```python
from build123d import *

# Parameters (mm, degrees)
F0_R     = 23.495
F0_R_2   = 19.05
F1_DEPTH = 6.35
F2_DEPTH = 149.86
F4_D     = 3.4544
F4_DEPTH = 12.7
F4_TIP   = 1.0378064612
F7_R     = 11.90625
F8_DEPTH = 0.381


with BuildPart() as f1:
    # F0 (on Top) → F1 (new body)
    with BuildSketch(Plane.XY):
        Circle(F0_R)
        Circle(F0_R_2, mode=Mode.SUBTRACT)
    extrude(amount=F1_DEPTH)

    # F0 (on Top) → F2 (join)
    with BuildSketch(Plane.XY):
        Circle(F0_R_2)
    extrude(amount=F2_DEPTH)

    # F4
    with Locations(Plane.XY.offset(149.86)):
        with Locations((0, 0)):
            Hole(F4_D / 2, depth=F4_DEPTH)
            with Locations((0, 0, -(F4_DEPTH + F4_TIP / 2))):  # 118° drill point
                Cone(0, F4_D / 2, F4_TIP, mode=Mode.SUBTRACT)


with BuildPart() as f5_1:
    # F5: copy of F1
    add(f1.part)


with BuildPart() as f1_1:
    add(f1.part)

    # F7 (on face) → F8 (cut)
    with BuildSketch(Plane(origin=(0, 0, 0), x_dir=(1, 0, 0), z_dir=(0, 0, -1))):
        Circle(F7_R)
    extrude(amount=-F8_DEPTH, mode=Mode.SUBTRACT)


solid = f1_1.part
```
Model file for the job. Use its own axes, mm. A direction names the side the tool comes from. Coordinates: 2 decimals unless noted, no trailing zeros. Order: outer loops, then holes, each group sorted by start corner. A loop starts at its lowest first (then second) coordinate and runs counter-clockwise, first axis right, second up. Notation, with made-up numbers: (38, 75) -> (60, 75) arc R4 ccw to (60, 79) -> close; hole circle Ø9 at (68, 29). An arc over 180 degrees is marked (long way). Answer as a JSON object with one key per item and string values. Group by question number.
1) Cut at A-A, the plane y = 8.5. Write the cut outline in (x, z).
2) Drill centre lines: L1, parallel to Y at x = 0, z = 144; L2, parallel to Y at x = 0, z = 0.1 (3 decimals); L3, parallel to Z at x = 19.5, y = -6. Where is each one in solid material? Low to high.
3) Pull direction X, two halves, no side cores. Call faces 4 (the face through (-15.12, -11.59, 77.1)), 5 (the face through (0, 0, 0.381)), 6 (the face through (-11, 6, 0)): +X half, -X half, draft (parallel to the pull), parting line (faces both ways), or undercut.
4) Which spindle directions (+Z, -Z, +X, -X, +Y, -Y) get a long thin tool onto all of the face, cutting with end or side? Do faces 1 (the face through (-5.093, -22.936, 3.131)), 2 (the face through (-0.1, 19.3, 6.35)), 3 (the face through (-9.45, 7.24, 0.19)). Say none if no direction does.
5) Cut at C-C, the plane z = 35. Write the cut outline in (x, y).
6) Flat gauge pins, fed straight in: pin 1 (5 mm diameter, centred on y = -14.5, z = 89.5, fed in from +X); pin 2 (5 mm diameter, centred on x = 9.5, z = 33, fed in from -Y); pin 3 (3 mm diameter, centred on y = 14.5, z = 122, fed in from +X). Where does each tip first touch, or does it go through?
7) Cut at D-D, the plane y = 14.5. Write the cut outline in (x, z), then the cut area to 3 significant figures.
8) Cut at B-B, the plane x = -14. Write the cut outline in (y, z).
Check values:
{
 "1": {"outline": "(-21.9, 0) -> (-8.34, 0) -> (-8.34, 0.38) -> (8.34, 0.38) -> (8.34, 0) -> (21.9, 0) -> (21.9, 6.35) -> (17.05, 6.35) -> (17.05, 149.86) -> (-17.05, 149.86) -> (-17.05, 6.35) -> (-21.9, 6.35) -> close"},
 "2": {"L1": "y = -19.05 to -1.73, 1.73 to 19.05", "L2": "y = -23.495 to -11.906, 11.906 to 23.495", "L3": "z = 0 to 6.35"},
 "3": {"face 4": "parting line", "face 5": "undercut", "face 6": "draft"},
 "4": {"face 1": "+Z, -Z", "face 2": "+Z", "face 3": "-Z"},
 "5": {"outline": "circle Ø38.1 at (0, 0)"},
 "6": {"pin 1": "stops at x = 14.8", "pin 2": "stops at y = -17.72", "pin 3": "stops at x = 13.92"},
 "7": {"outline": "(-18.49, 0) -> (18.49, 0) -> (18.49, 6.35) -> (12.36, 6.35) -> (12.36, 149.86) -> (-12.36, 149.86) -> (-12.36, 6.35) -> (-18.49, 6.35) -> close", "area": "3,780 mm²"},
 "8": {"outline": "(-18.87, 0) -> (18.87, 0) -> (18.87, 6.35) -> (12.92, 6.35) -> (12.92, 149.86) -> (-12.92, 149.86) -> (-12.92, 6.35) -> (-18.87, 6.35) -> close"}
}
